The drawing under review shows one solid part. Ordinate dimensions are in mm from its lowest x, y, z. Coordinates: 2 decimals unless noted, no trailing zeros. Loops run counter-clockwise (first coordinate to the right, second up) from the corner with the lowest first, then second, coordinate; pieces in that order, holes last. Notation, with made-up numbers: (-19, 17) -> (-4, 17) arc R11 cw to (-4, 22) -> close; hole circle Ø9 at (19.25, -29.75). An arc over 180 degrees is marked (long way). Use a Markdown table: item, result.
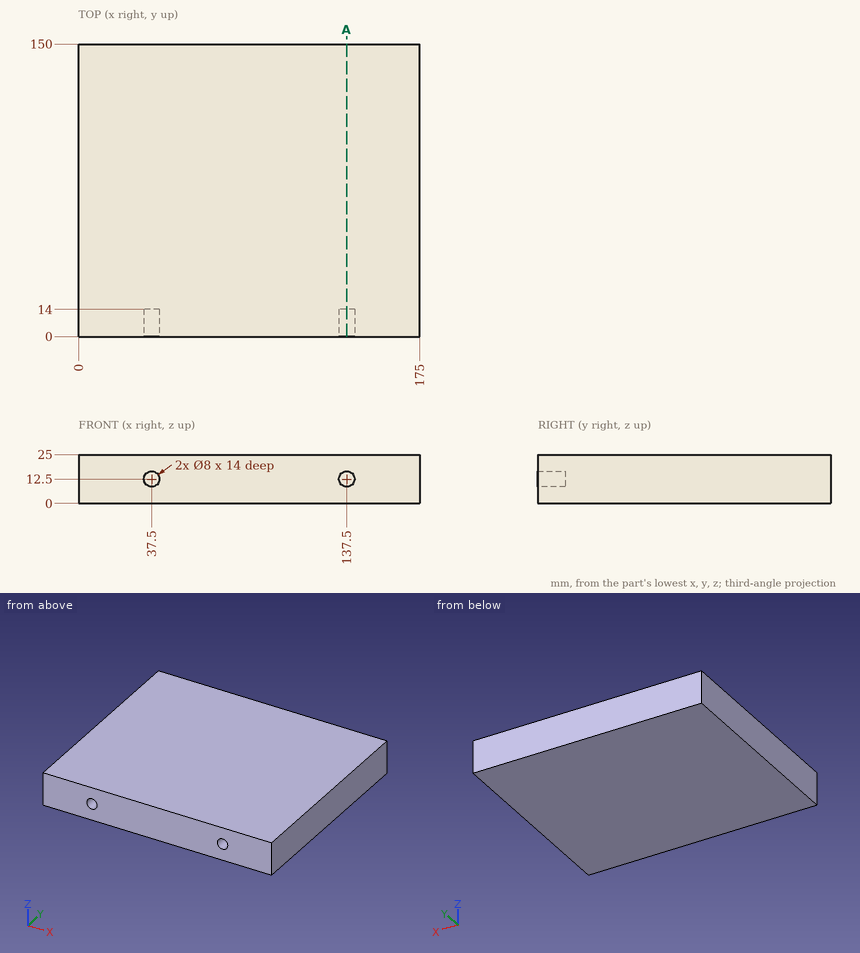
(1) For pin 1 Ø2 at (x, y) = (140, 41) entering from -Z; pin 2 Ø2.5 at (x, z) = (137, 14) entering from -Y, all flat-tipped, find the tip position at first contact; note any pin that passes through.
Found:
| item | result |
|---|---|
| pin 1 | stops at z = 0 |
| pin 2 | stops at y = 14 |
(2) For line 1 along X through (y, z) = (6, 12.5); line 2 along Z through (x, y) = (137, 8); line 3 along Y through (x, z) = (136.5, 9), list the stretches that pass through material, from the lowest coordinate up.
Found:
| item | result |
|---|---|
| line 1 | x = 0 to 33.5, 41.5 to 133.5, 141.5 to 175 |
| line 2 | z = 0 to 8.53, 16.47 to 25 |
| line 3 | y = 14 to 150 |
(3) Take a section at A-A on x = 137.5. Write out the cut boundary in (y, z), plus the area to 3 significant figures.
Found:
| item | result |
|---|---|
| outline | (0, 0) -> (150, 0) -> (150, 25) -> (0, 25) -> (0, 16.5) -> (14, 16.5) -> (14, 8.5) -> (0, 8.5) -> close |
| area | 3,640 mm^2 |
